```python
from build123d import *

# Parameters (mm, degrees)
BOSS_EXTRUDE1_DEPTH     = 101.6
SKETCH2_W               = 19.05
SKETCH2_H               = 15.875
CUT_EXTRUDE1_DEPTH      = 6.35
SKETCH3_W               = 19.05
SKETCH3_H               = 15.875
CUT_EXTRUDE2_DEPTH      = 6.35
SKETCH4_R               = 1.3890625
CUT_EXTRUDE3_DEPTH      = 1
CUT_EXTRUDE3_DEPTH_BACK = 16.875


with BuildPart() as part:
    # Sketch1 → Boss-Extrude1 (new body, symmetric)
    with BuildSketch(Plane.XY):
        Polygon((-9.525, 12.7), (-3.175, 12.7), (-3.175, 0), (3.175, 0), (3.175, 12.7), (9.525, 12.7), (9.525, -3.175), (-9.525, -3.175), align=None)
    extrude(amount=BOSS_EXTRUDE1_DEPTH, both=True)

    # Sketch2 → Cut-Extrude1 (cut)
    with BuildSketch(Plane.XY.offset(-101.6)):
        with Locations((0, 4.7625)):
            Rectangle(SKETCH2_W, SKETCH2_H)
    extrude(amount=CUT_EXTRUDE1_DEPTH, mode=Mode.SUBTRACT)

    # Sketch3 → Cut-Extrude2 (cut)
    with BuildSketch(Plane(origin=(0, 0, -95.25), x_dir=(-1, 0, 0), z_dir=(0, 0, -1))):
        with Locations((0, 4.7625)):
            Rectangle(SKETCH3_W, SKETCH3_H)
    extrude(amount=-CUT_EXTRUDE2_DEPTH, mode=Mode.SUBTRACT)

    # Sketch4 → Cut-Extrude3 (cut, two sides)
    with BuildSketch(Plane(origin=(0, 12.7, 0), x_dir=(1, 0, 0), z_dir=(0, 1, 0))) as cut_extrude3_sk:
        with Locations((6.35, 85.725)):
            Circle(SKETCH4_R)
        with Locations((-6.35, 85.725)):
            Circle(SKETCH4_R)
        with Locations((6.35, -6.35)):
            Circle(SKETCH4_R)
        with Locations((-6.35, -6.35)):
            Circle(SKETCH4_R)
        with Locations((6.35, -98.425)):
            Circle(SKETCH4_R)
        with Locations((-6.35, -98.425)):
            Circle(SKETCH4_R)
    extrude(amount=CUT_EXTRUDE3_DEPTH, mode=Mode.SUBTRACT)
    extrude(cut_extrude3_sk.sketch, amount=-CUT_EXTRUDE3_DEPTH_BACK, mode=Mode.SUBTRACT)


solid = part.part
```
The listing builds one solid part. Answer for the finished solid, in the listing's coordinates (mm). A direction names the side the tool comes from. Round coordinates to 2 decimals unless told otherwise and drop trailing zeros. Write each loop counter-clockwise with the first axis right and the second up, starting at its lowest first coordinate (ties: lowest second). Pieces come first, ordered by that corner, then holes. Notation, with made-up numbers: (48, 64.25) -> (90, 64.25) arc R23 ccw to (90, 87.25) -> close; hole circle Ø10 at (61.5, 25.25). An arc over 180 degrees is marked (long way). Answer as a JSON object with one key per item and string values. Group by question number.
Q1. Section C-C (x = 1) is taken. Write down the section's boundary in (y, z) (3 decimals), plus the area to 3 significant figures.
Q2. Which of the six approach directions +Z, -Z, +X, -X, +Y, -Y give full straight-line access (tool end or side, diameter ignored) to faces 1 (the face through (0, -3.175, 8)), 2 (the face through (-3.175, 6, 8))?
Q3. Straight lines are drawn through the part: line 1 along Z through (x, y) = (-6.35, 0.75); line 2 along X through (y, z) = (5, -73.5) (3 decimals); line 3 along Z through (x, y) = (-6.75, 1.5). For each, find the intervals that lie inside material, in ascending order.
Q4. Determine the mould class of faces 3 (the face through (3.175, 6, 8)), 4 (the face through (9.525, 5, 8)), 5 (the face through (-4, 5, 101.6)) for opening direction X: pulls with the +X half, pulls with the -X half, needs draft (parallel to the pull), parting line crosses it, or undercut.
Q5. Section A-A (y = 10) is taken. Write down the section's boundary in (x, z) (3 decimals), plus the area to 3 significant figures.
Q6. Section B-B (z = 72.5) is taken. Write down the section's boundary in (x, y) (3 decimals).
Check values:
{
 "1": {"outline": "(-3.175, -88.9) -> (0, -88.9) -> (0, 101.6) -> (-3.175, 101.6) -> close", "area": "605 mm^2"},
 "2": {"face 1": "+Z, -Z, +X, -X, -Y", "face 2": "+Z, -Z, +Y"},
 "3": {"line 1": "-88.9 to -87.11, -84.34 to 4.96, 7.74 to 97.04, 99.81 to 101.6", "line 2": "-9.525 to -3.175, 3.175 to 9.525", "line 3": "-88.9 to -87.06, -84.39 to 5.02, 7.68 to 97.09, 99.76 to 101.6"},
 "4": {"face 3": "undercut", "face 4": "pulls with the +X half", "face 5": "needs draft"},
 "5": {"outline": "(-9.525, -88.9) -> (-3.175, -88.9) -> (-3.175, 101.6) -> (-9.525, 101.6) -> close; (3.175, -88.9) -> (9.525, -88.9) -> (9.525, 101.6) -> (3.175, 101.6) -> close; hole circle Ø2.778 at (-6.35, -85.725); hole circle Ø2.778 at (-6.35, 6.35); hole circle Ø2.778 at (-6.35, 98.425); hole circle Ø2.778 at (6.35, -85.725); hole circle Ø2.778 at (6.35, 6.35); hole circle Ø2.778 at (6.35, 98.425)", "area": "2,380 mm^2"},
 "6": {"outline": "(-9.525, -3.175) -> (9.525, -3.175) -> (9.525, 12.7) -> (3.175, 12.7) -> (3.175, 0) -> (-3.175, 0) -> (-3.175, 12.7) -> (-9.525, 12.7) -> close"}
}
